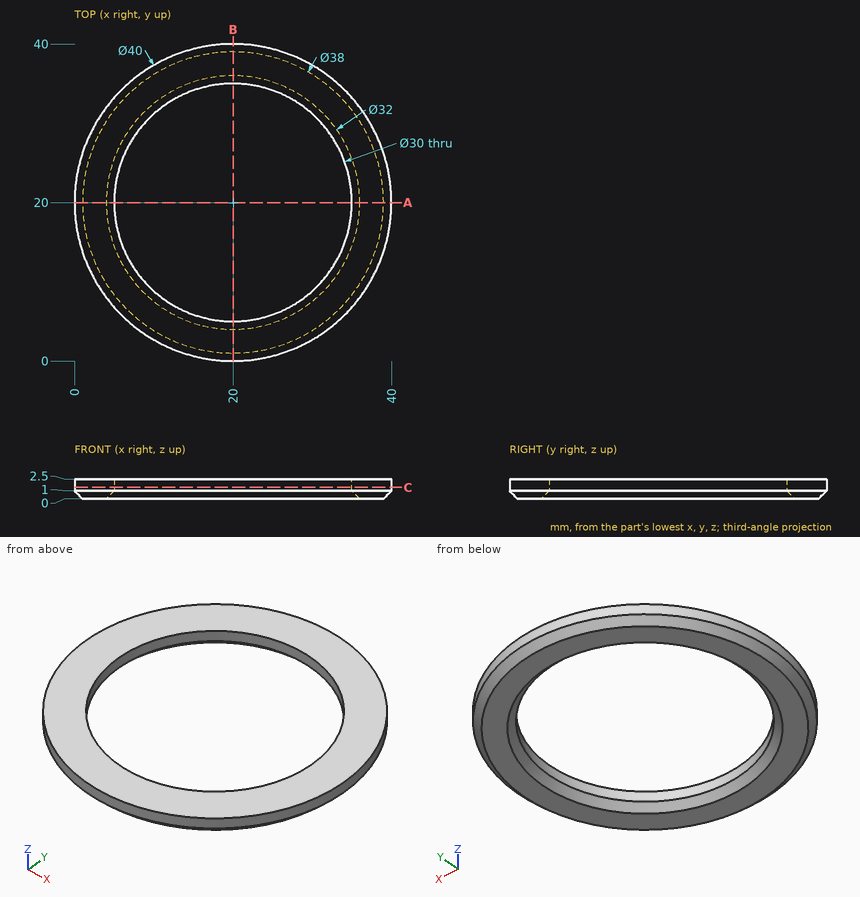
For this review, use the dimensioned drawing (mm, ordinates from the lowest corner) and the shaded views. Round coordinates to 2 decimals unless told otherwise and drop trailing zeros. Write each loop counter-clockwise with the first axis right and the second up, starting at its lowest first coordinate (ties: lowest second). Pieces come first, ordered by that corner, then holes. Notation, with made-up numbers: M 86,19 L 94,19 A7 cw 94,31 Z; hole C -27,25.25 d7. An arc over 180 degrees is marked long. Use CSV: the item, a comma, the result in double quotes. Start each with the question number.
(1) We need section A-A, the plane y = 20. State the section outline as (x, z) points, then the cut area to 3 significant figures.
(2) We need section C-C, the plane z = 1.45. State the section outline as (x, y) points, then the cut area to 3 significant figures.
(3) Clearance check with flat-ended pins moving along their axes: P1, Ø1.5, axis at x = 22, z = 0.5, coming from the -Y side; P2, Ø1.5, axis at x = 33.5, y = 14.5, coming from the +Z side. State where each tip first meets the part, or that it passes through.
(4) For line 1 along Y through (x, z) = (20, 1.5); line 2 along X through (y, z) = (33, 1.6); line 3 along Y through (x, z) = (9, 1.8), list the stretches that pass through material, from the lowest coordinate up.
Findings:
1,outline,"M 0,1 L 1,0 L 4,0 L 5,1 L 5,2.5 L 0,2.5 Z; M 35,1 L 36,0 L 39,0 L 40,1 L 40,2.5 L 35,2.5 Z"
1,area,"23.0 mm^2"
2,outline,"C 20,20 d40; hole C 20,20 d30"
2,area,"550 mm^2"
3,P1,"y = 0.05"
3,P2,"z = 2.5"
4,line 1,"0 to 5, 35 to 40"
4,line 2,"4.8 to 12.52, 27.48 to 35.2"
4,line 3,"3.3 to 9.8, 30.2 to 36.7"
